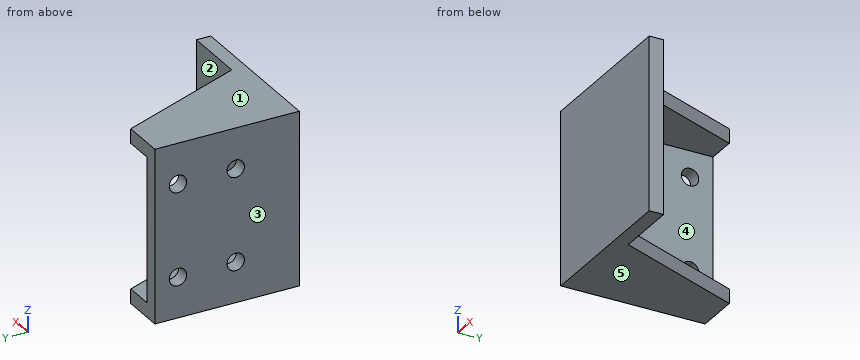
from build123d import *

# Parameters (mm, degrees)
EXTRUDE_1_DEPTH     = 60
SKETCH_2_W          = 34.644902364
SKETCH_2_H          = 50
CUT_EXTRUDE_1_DEPTH = 45
SKETCH_3_R          = 3
SKETCH_3_R_2        = 2.5
CUT_EXTRUDE_2_DEPTH = 91.891477881
SKETCH_4_R          = 3
CUT_EXTRUDE_3_DEPTH = 82.627431502
SKETCH_5_W          = 60
SKETCH_5_H          = 5
EXTRUDE_2_DEPTH     = 50


with BuildPart() as part:
    # 草图1 → 凸台-拉伸1 (new body)
    with BuildSketch(Plane.XY):
        Polygon((-11.489361702, -7.127659574), (-46.489361702, -7.127659574), (-46.489361702, 42.872340426), (-31.489361702, 42.872340426), align=None)
    extrude(amount=EXTRUDE_1_DEPTH)

    # 草图2 → 切除-拉伸1 (cut)
    with BuildSketch(Plane(origin=(0, 42.872340426, 0), x_dir=(1, 0, 0), z_dir=(0, 1, 0))):
        with Locations((-24.16691052, -30)):
            Rectangle(SKETCH_2_W, SKETCH_2_H)
    extrude(amount=-CUT_EXTRUDE_1_DEPTH, mode=Mode.SUBTRACT)

    # 草图3 → 切除-拉伸2 (cut, through all)
    with BuildSketch(Plane.XZ.offset(7.127659574)):
        with Locations((-35.489361702, 48)):
            Circle(SKETCH_3_R)
        with Locations(Location((-35.489361702, 12, 0), (0, 0, 270))):
            Circle(SKETCH_3_R)
        with Locations(Location((-19.489361702, 12, 0), (0, 0, 270))):
            Circle(SKETCH_3_R_2)
        with Locations((-19.489361702, 48)):
            Circle(SKETCH_3_R_2)
    extrude(amount=-CUT_EXTRUDE_2_DEPTH, mode=Mode.SUBTRACT)

    # 草图4 → 切除-拉伸3 (cut, through all)
    with BuildSketch(Plane.ZY.offset(46.489361702)):
        with Locations((14, 34.872340426)):
            Circle(SKETCH_4_R)
        with Locations((46, 34.872340426)):
            Circle(SKETCH_4_R)
        with Locations((14, 14.872340426)):
            Circle(SKETCH_4_R)
        with Locations((46, 14.872340426)):
            Circle(SKETCH_4_R)
    extrude(amount=-CUT_EXTRUDE_3_DEPTH, mode=Mode.SUBTRACT)

    # 草图5 → 凸台-拉伸2 (add)
    with BuildSketch(Plane(origin=(-41.489361702, 0, 0), x_dir=(0, 0, -1), z_dir=(1, 0, 0))):
        with Locations((-30, -4.627659574)):
            Rectangle(SKETCH_5_W, SKETCH_5_H)
    extrude(amount=EXTRUDE_2_DEPTH)


solid = part.part
Geometry check sheet. Reference: the model listing, model coordinates, mm. Face numbers are marked on the shaded views. A direction names the side the tool comes from. Coordinates: 2 decimals unless noted, no trailing zeros. Order: outer loops, then holes, each group sorted by start corner. A loop starts at its lowest first (then second) coordinate and runs counter-clockwise, first axis right, second up. Notation, with made-up numbers: (70, -3.5) - (122, -3.5) arc R7 cw to (122, 0.5) - close; hole circle Ø6 at (-18.75, 83). An arc over 180 degrees is marked (long way). Answer in a Markdown table with one row per item. Add a question column.
1) Release check for a two-part mould opening along Z. For the marked faces 3, 4 and 5 record: +Z half, -Z half, draft (parallel to the pull), parting line (faces both ways), or undercut.
2) Cross-section at C-C, the plane y = 14. Record the cut outline in (x, z), then the cut area to 3 significant figures.
3) Gauge pin test, flat ends, axial feed: P1, Ø7, axis at y = 14.87, z = 14, coming from the +X side; P2, Ø1, axis at x = -10.5, z = 23, coming from the +Y side. Record the tip position at first contact, or that the pin passes through.
4) Cross-section at D-D, the plane z = 21. Record the cut outline in (x, y), then the cut area to 3 significant figures.
5) Cross-section at A-A, the plane z = 46. Record the cut outline in (x, y).
6) Set-up check for the marked faces 1 and 2: record each of +Z, -Z, +X, -X, +Y, -Y from which the full face is reachable in a straight line by a thin tool's end or side.
7) Material ranges on line 1 along Y through (x, z) = (-43, 46); line 2 along Z through (x, y) = (-26, 16); line 3 along Y through (x, z) = (-43.5, 16.5), recorded low to high. Write a range as [from, to].
8) Cross-section at B-B, the plane x = -42.5. Record the cut outline in (y, z), then the cut area to 3 significant figures.
Check result:
| question | item | result |
|---|---|---|
| 1 | face 3 | draft |
| 1 | face 4 | undercut |
| 1 | face 5 | -Z half |
| 2 | outline | (-46.49, 0) - (-19.94, 0) - (-19.94, 5) - (-41.49, 5) - (-41.49, 11.13) - (-46.49, 11.13) - close; (-46.49, 16.87) - (-41.49, 16.87) - (-41.49, 43.13) - (-46.49, 43.13) - close; (-46.49, 48.87) - (-41.49, 48.87) - (-41.49, 55) - (-19.94, 55) - (-19.94, 60) - (-46.49, 60) - close |
| 2 | area | 458 mm² |
| 3 | P1 | stops at x = -41.49 |
| 3 | P2 | stops at y = -2.13 |
| 4 | outline | (-46.49, -7.13) - (8.51, -7.13) - (8.51, -2.13) - (-41.49, -2.13) - (-41.49, 42.87) - (-46.49, 42.87) - close |
| 4 | area | 500 mm² |
| 5 | outline | (-46.49, -7.13) - (8.51, -7.13) - (8.51, -2.13) - (-41.49, -2.13) - (-41.49, 11.87) - (-46.49, 11.87) - close; (-46.49, 17.87) - (-41.49, 17.87) - (-41.49, 31.87) - (-46.49, 31.87) - close; (-46.49, 37.87) - (-41.49, 37.87) - (-41.49, 42.87) - (-46.49, 42.87) - close |
| 6 | face 1 | +Z, +X, -X, +Y, -Y |
| 6 | face 2 | +X, +Y |
| 7 | line 1 | y = [-7.13, 11.87], [17.87, 31.87], [37.87, 42.87] |
| 7 | line 2 | z = [0, 5], [55, 60] |
| 7 | line 3 | y = [-7.13, 13.21], [16.53, 33.21], [36.53, 42.87] |
| 8 | outline | (-7.13, 0) - (42.87, 0) - (42.87, 60) - (-7.13, 60) - close; hole circle Ø6 at (14.87, 14); hole circle Ø6 at (14.87, 46); hole circle Ø6 at (34.87, 14); hole circle Ø6 at (34.87, 46) |
| 8 | area | 2,890 mm² |
